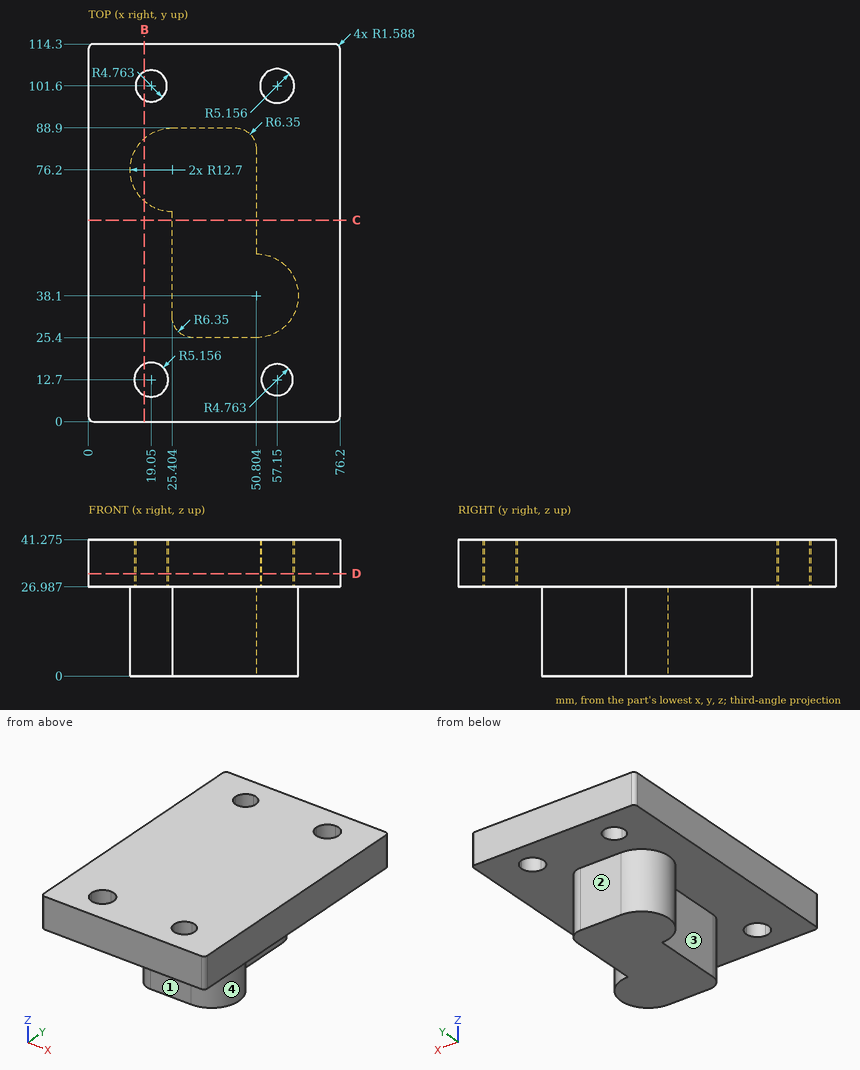
Geometry check sheet. Reference: drawing and pictorial views, mm from the part's lowest x, y, z. A direction names the side the tool comes from. Give positions to 0.01 mm unless a question says otherwise; leave off trailing zeros. Write each loop counter-clockwise with the first axis right and the second up, starting at its lowest first coordinate (ties: lowest second). Pieces come first, ordered by that corner, then holes. Notation, with made-up numbers: (61.5, 67) -> (76.5, 67) arc R9 ccw to (76.5, 79) -> close; hole circle Ø11 at (78, -7). An arc over 180 degrees is marked (long way). One line per question, with ' | ' between items.
Item 1: Sectioned sample at B-B, the plane x = 17. Record the boundary of the cut face in (y, z) (1 decimal), plus the area to 3 significant figures.
Determined:
outline: (0, 27) -> (8, 27) -> (8, 41.3) -> (0, 41.3) -> close; (17.4, 27) -> (66.7, 27) -> (66.7, 0) -> (85.7, 0) -> (85.7, 27) -> (97.3, 27) -> (97.3, 41.3) -> (17.4, 41.3) -> close; (105.9, 27) -> (114.3, 27) -> (114.3, 41.3) -> (105.9, 41.3) -> close | area: 1,890 mm^2
Item 2: Access from +Z, -Z, +X, -X, +Y, -Y to the whole of each face (thin tool, end or side, straight path). Record for the marked faces 1, 2, 3 and 4.
Determined:
face 1: -Z, +X, -X, -Y | face 2: -Z, +X, -X, +Y | face 3: -Z, -X, -Y | face 4: -Z, +X
Item 3: Depth check by flat-ended pin: pin 1 (5.5 mm diameter, centred on x = 31, z = 14.5, fed in from +Y); pin 2 (1.5 mm diameter, centred on y = 79, z = 25.5, fed in from -X); pin 3 (10 mm diameter, centred on x = 66, y = 27, fed in from -Z). Enter the tip coordinate at first touch or a pass-through.
Determined:
pin 1: y = 88.9 | pin 2: x = 12.87 | pin 3: z = 26.99
Item 4: Scan lines: line 1 along Y through (x, z) = (21.5, 38.5) (1 decimal); line 2 along Y through (x, z) = (18, 29) (1 decimal); line 3 along Z through (x, y) = (22, 37.5) (1 decimal). Record each from-to range of solid material in increasing order.
Determined:
line 1: 0 to 8.2, 17.2 to 97.5, 105.7 to 114.3 | line 2: 0 to 7.7, 17.7 to 97, 106.2 to 114.3 | line 3: 27 to 41.3
Item 5: Sectioned sample at C-C, the plane y = 61. Record the boundary of the cut face in (x, z) (1 decimal).
Determined:
outline: (0, 27) -> (25.4, 27) -> (25.4, 0) -> (50.8, 0) -> (50.8, 27) -> (76.2, 27) -> (76.2, 41.3) -> (0, 41.3) -> close
Item 6: Sectioned sample at D-D, the plane z = 31. State how many separate pieces and enclosed holes the cut face has, plus the area to 3 significant figures.
Determined:
separate pieces: 1 | enclosed holes: 4 | area: 8,400 mm^2
